Geometry: see drawing. Coordinates: mm, zero at the bounding-box minimum. A direction names the side the tool comes from. Give positions to 0.01 mm unless a question says otherwise; leave off trailing zeros. Write each loop counter-clockwise with the first axis right and the second up, starting at its lowest first coordinate (ties: lowest second). Pieces come first, ordered by that corner, then holes. Notation, with made-up numbers: M 38,9.25 L 45,9.25 A20 ccw 45,35.25 Z; hole C 26,39 d9. An arc over 180 degrees is marked long. Use a Markdown table: item, result. Add a question column.
1) Section D-D on x = 68. Return the cut outline in (y, z).
2) Section A-A on z = 18. Return the cut outline in (x, y).
3) Section C-C on y = 11. Return the cut outline in (x, z), then the cut area to 3 significant figures.
4) Section B-B on x = 76. Return the cut outline in (y, z).
5) Draft query along X for the marked faces 3 and 4. Return one class per face: +X half, -X half, draft (parallel to the pull), parting line (faces both ways), or undercut.
6) Line query: line 1 (Z direction, x = 52.5, y = 10.25); line 2 (Y direction, x = 19.5, z = 2); line 3 (X direction, y = 18.5, z = 2.5). Output: solid intervals per line, ascending.
7) Set-up query: the marked faces 1 and 2. Return all of +Z, -Z, +X, -X, +Y, -Y with unobstructed straight access to the full face (end or side cutting, diameter ignored); none if empty.
8) Pin query (flat end, axial travel): pin 1 (4 mm diameter, centred on x = 78, z = 18, fed in from +Y); pin 2 (1.2 mm diameter, centred on x = 8, z = 2.5, fed in from -Y); pin 3 (1.2 mm diameter, centred on y = 17.5, z = 1, fed in from +X). Return the tip coordinate at first contact, or that it passes through.
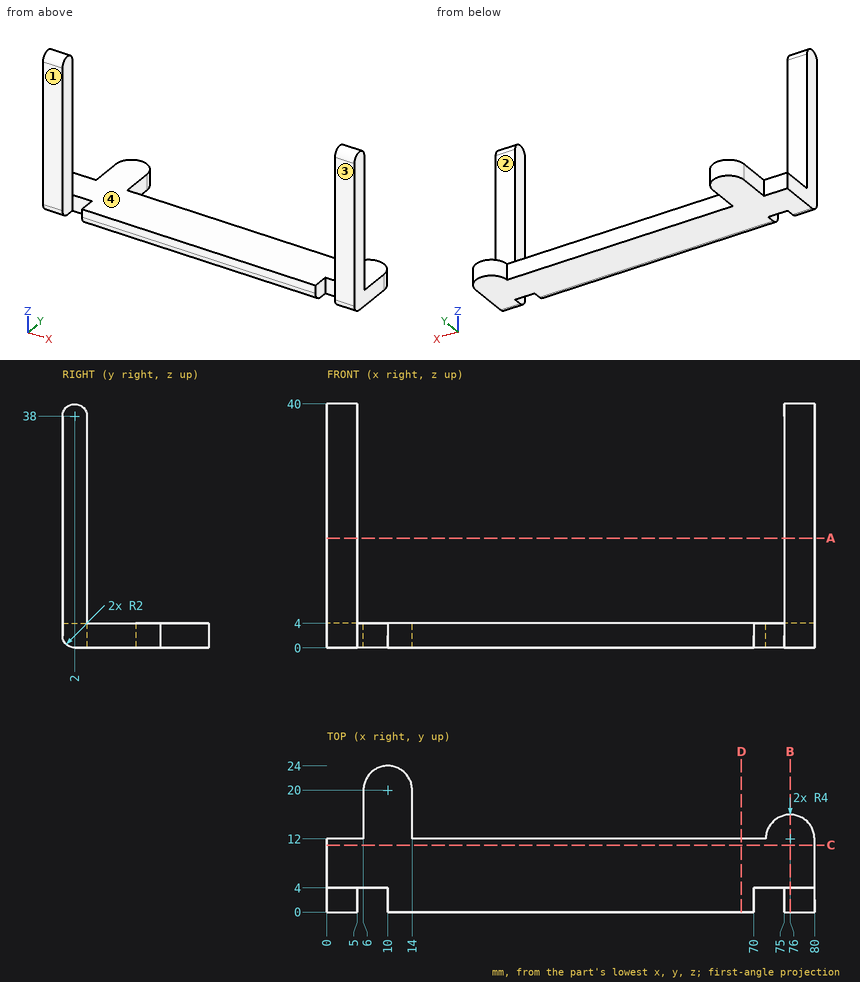
Found:
| question | item | result |
|---|---|---|
| 1 | outline | M 0,2 A2 ccw 2,0 L 12,0 L 12,4 L 0,4 Z |
| 2 | outline | M 0,0 L 5,0 L 5,4 L 0,4 Z; M 75,0 L 80,0 L 80,4 L 75,4 Z |
| 3 | outline | M 0,0 L 80,0 L 80,4 L 0,4 Z |
| 3 | area | 320 mm² |
| 4 | outline | M 0,2 A2 ccw 2,0 L 16,0 L 16,4 L 4,4 L 4,38 A2 ccw 0,38 Z |
| 5 | face 3 | draft |
| 5 | face 4 | undercut |
| 6 | line 1 | 0 to 4 |
| 6 | line 2 | 0 to 12 |
| 6 | line 3 | 6 to 14 |
| 7 | face 1 | +Z, -Z, +X, -X, -Y |
| 7 | face 2 | +Z, +X, -X, +Y |
| 8 | pin 1 | y = 4 |
| 8 | pin 2 | y = 4 |
| 8 | pin 3 | x = 14 |
